from build123d import *

# Parameters (mm, degrees)
SKETCH1_R           = 4
BOSS_EXTRUDE1_DEPTH = 2
SKETCH2_R           = 1.95
BOSS_EXTRUDE2_DEPTH = 14
CHAMFER1_SIZE       = 2
CUT_EXTRUDE1_DEPTH  = 1.5


with BuildPart() as part:
    # Sketch1 → Boss-Extrude1 (new body)
    with BuildSketch(Plane(origin=(0, 0, 0), x_dir=(1, 0, 0), z_dir=(0, 1, 0))):
        with Locations(Location((0, 0, 0), (0, 0, 270))):
            Circle(SKETCH1_R)
    extrude(amount=BOSS_EXTRUDE1_DEPTH)

    # Sketch2 → Boss-Extrude2 (add)
    with BuildSketch(Plane(origin=(0, 2, 0), x_dir=(1, 0, 0), z_dir=(0, 1, 0))):
        with Locations(Location((0, 0, 0), (0, 0, 270))):
            Circle(SKETCH2_R)
    extrude(amount=BOSS_EXTRUDE2_DEPTH)

    # Chamfer1
    chamfer1_edges = [part.edges().sort_by_distance(p)[0] for p in [
        (0, 2, -4),
    ]]
    chamfer(chamfer1_edges, length=CHAMFER1_SIZE - 0.0001)  # a hair under: the kernel refuses the full size

    # Sketch3 → Cut-Extrude1 (cut)
    with BuildSketch(Plane.XZ):
        Polygon((0, -1.662470902), (1.439742034, -0.831235451), (1.439742034, 0.831235451), (0, 1.662470902), (-1.439742034, 0.831235451), (-1.439742034, -0.831235451), align=None)
    extrude(amount=-CUT_EXTRUDE1_DEPTH, mode=Mode.SUBTRACT)


solid = part.part
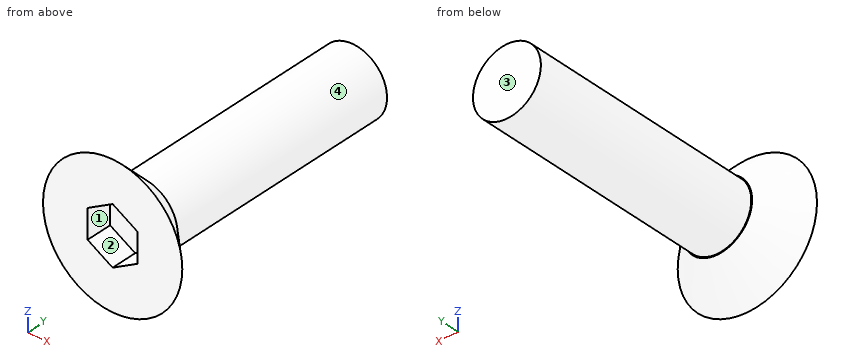
Check sheet for the modelled part. Datum: model origin and axes. Units: mm. Face numbers are marked on the shaded views. Round coordinates to 2 decimals unless told otherwise and drop trailing zeros. Order: outer loops, then holes, each group sorted by start corner. A loop starts at its lowest first (then second) coordinate and runs counter-clockwise, first axis right, second up.
(1) Cross-section at C-C, the plane y = 1.75. Enter the section's corners in (x, z).
(2) Cross-section at B-B, the plane y = 10.5. Enter the section's corners in (x, z).
(3) Draft check along X on the marked faces 1, 2, 3 and 4. Enter one of: pulls with the +X half, pulls with the -X half, needs draft (parallel to the pull), parting line crosses it, or undercut.
(4) Go/stop test with flat-tipped pins: P1, Ø4, axis at x = 2.5, z = 2, coming from the -Y side; P2, Ø1.5, axis at x = 1.5, z = -2.5, coming from the +Y side; P3, Ø1.2, axis at y = 1, z = 0, coming from the +X side; P4, Ø2, axis at x = -2.5, y = 7, coming from the -Z side. Record where each tip stops, or that it passes through.
(5) Scan lines: probe 1 along Y at (x, z) = (0.5, 0.25); probe 2 along X at (y, z) = (1, -0.5); probe 3 along Y at (x, z) = (1.75, 3). Record each from-to range of solid material in increasing order.
Check sheet entries:
1. outline: circle Ø4.5 at (0, 0)
2. outline: circle Ø3.9 at (0, 0)
3. face 1: undercut
3. face 2: undercut
3. face 3: needs draft
3. face 4: parting line crosses it
4. P1: stops at y = 0
4. P2: stops at y = 1.83
4. P3: stops at x = 3.6
4. P4: stops at z = -1.25
5. probe 1: y = 1.5 to 16
5. probe 2: x = -2.96 to -1.44, 1.44 to 2.96
5. probe 3: y = 0 to 0.53
